Source: CAD feature listing. Evaluate the final solid. Frame: model axes, mm. Face numbers are marked on the shaded views. A direction names the side the tool comes from. Round coordinates to 2 decimals unless told otherwise and drop trailing zeros. Write each loop counter-clockwise with the first axis right and the second up, starting at its lowest first coordinate (ties: lowest second). Pieces come first, ordered by that corner, then holes. Notation, with made-up numbers: (60, 74.5) - (110, 74.5) arc R16 cw to (110, 80.5) - close; hole circle Ø1 at (9, 59). An arc over 180 degrees is marked (long way). Write item = value, one per line. Start each with the question number.
Autodesk Inventor part; units mm, degrees
ref_plane "YZ Plane" through (0, 0, 0) normal (1, 0, 0) x (0, 1, 0)
ref_plane "XZ Plane" through (0, 0, 0) normal (0, 1, 0) x (-1, 0, 0)
ref_plane "XY Plane" through (0, 0, 0) normal (0, 0, 1) x (1, 0, 0)
sketch "Sketch1" plane through (0, 0, 0) normal (1, 0, 0) x (0, 1, 0)
  line L0 (0, 50) -> (0, -50)
  line L1 (0, -50) -> (5, -50)
  line L2 (5, -50) -> (5, -37)
  line L3 (5, -37) -> (17.41, -37)
  line L4 (24, -30.41) -> (24, 30.41)
  line L5 (17.41, 37) -> (5, 37)
  line L6 (5, 37) -> (5, 50)
  line L7 (5, 50) -> (0, 50)
  line L8 (21.5, 11) -> (13.5, 11)
  line L9 (13.5, 11) -> (13.5, -17)
  line L10 (13.5, -17) -> (21.5, -17)
  line L11 (21.5, -17) -> (21.5, 11)
  circle A0 centre (11.9411, 30) radius 4
  circle A1 centre (11.9411, -30) radius 4
  arc A2 (24, 30.41) -> (17.41, 37) centre (17.41, 30.41) ccw
  arc A3 (17.41, -37) -> (24, -30.41) centre (17.41, -30.41) ccw
  point P0 (0, 0)
  point P1 (24, -37)
  point P2 (0, 0)
  dimension "d0" = 100
  dimension "d1" = 5
  dimension "d2" = 13
  dimension "d3" = 13
  dimension "d4" = 19
  dimension "d5" = 28
  dimension "d6" = 26
  dimension "d7" = 8
  dimension "d8" = 2.5
  dimension "d9" = 8
  dimension "d10" = 60
  dimension "d11" = 30
  dimension "d12" = 6.59
extrude "Extrusion1" add sketch "Sketch1" along normal blind 12
sketch "Sketch2" plane through (0, 24, 30.41) normal (0, 1, 0) x (1, 0, 0)
  circle A0 centre (6, 33.41) radius 4
  line L0 (0, -6.59) -> (12, -6.59)
  point P0 (0, 30.41)
  point P1 (6, -6.59)
  dimension "d15" = 40
  dimension "d16" = 8
extrude "Extrusion2" cut sketch "Sketch2" against normal blind 20
sketch "Sketch3" plane through (0, 0, -50) normal (0, -1, 0) x (1, 0, 0)
  line L0 (4, 95) -> (4, 91)
  line L1 (8, 91) -> (8, 95)
  arc A0 (4, 91) -> (8, 91) centre (6, 91) ccw
  arc A1 (8, 95) -> (4, 95) centre (6, 95) ccw
  line L2 (0, 100) -> (12, 100)
  line L3 (0, 100) -> (0, 0)
  line L4 (4, 9) -> (4, 5)
  line L5 (8, 5) -> (8, 9)
  arc A2 (4, 5) -> (8, 5) centre (6, 5) ccw
  arc A3 (8, 9) -> (4, 9) centre (6, 9) ccw
  line L6 (0, 0) -> (12, 0)
  point P0 (0, 50)
  dimension "d19" = 4
  dimension "d20" = 4
  dimension "d21" = 5
  dimension "d22" = 6
  dimension "d23" = 4
  dimension "d24" = 4
  dimension "d25" = 5
extrude "Extrusion3" cut sketch "Sketch3" against normal up to next
sketch "Sketch5" plane through (0, 13.5, 11) normal (0, 1, 0) x (1, 0, 0)
  circle A0 centre (6, 14) radius 4
  circle A1 centre (6, 14) radius 5
  point P0 (0, 11)
  dimension "d28" = 10
extrude "Extrusion4" add sketch "Sketch5" along normal blind 0.5
pattern_linear "Rectangular Pattern1" count 2 spacing 7.5 along (0, 1, 0) of "Extrusion4"
equation "\"d3\" = d2"
properties material "ABS Plastic"
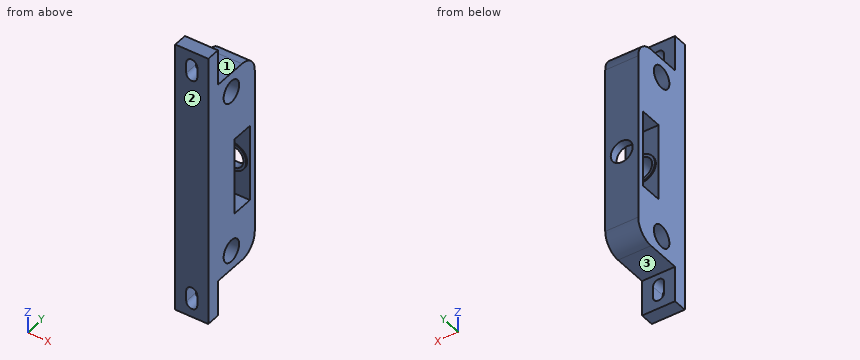
(1) Section C-C (x = 6). Count the separate pieces of the cut face and the enclosed holes in it, plus the area to 3 significant figures.
(2) Contact query for flat-ended pins moving along their axis: P1, Ø13, axis at y = 11.94, z = -30, coming from the -X side; P2, Ø6, axis at x = 8, y = 19, coming from the -Z side; P3, Ø4, axis at x = 6.5, y = 17.5, coming from the +Z side. Output: stop coordinate, or through.
(3) Section D-D (z = 32). Return the cut outline in (x, y).
(4) Section A-A (y = 10.25). Return the cut outline in (x, z), plus the area to 3 significant figures.
(5) Reachability of the marked faces 1, 2 and 3 from +Z, -Z, +X, -X, +Y, -Y: full face, straight path, thin tool, end or side. Return the list, or none.
(6) Section B-B (z = -3). Return the cut outline in (x, y).
(7) Ray query, L1, parallel to Z at x = 5.75, y = 4.5; L2, parallel to Z at x = 6, y = 8.5; L3, parallel to X at y = 22.25, z = -3. Return the intervals inside material, ascending. Write a range as from..to.
Solution:
q1.separate_pieces = 3
q1.enclosed_holes = 2
q1.area = 1,390 mm^2
q2.P1 = 0
q2.P2 = -37
q2.P3 = 37
q3.outline = (0, 0) - (12, 0) - (12, 8.48) - (0, 8.48) - close; (0, 15.41) - (12, 15.41) - (12, 23.81) - (0, 23.81) - close
q4.outline = (0, -37) - (12, -37) - (12, -33.62) - (0, -33.62) - close; (0, -26.38) - (12, -26.38) - (12, 26.38) - (0, 26.38) - close; (0, 33.62) - (12, 33.62) - (12, 37) - (0, 37) - close; hole circle Ø8 at (6, -3)
q4.area = 664 mm^2
q5.face_1 = +Z, +X, -X, +Y
q5.face_2 = +Z, -Z, +X, -X, -Y
q5.face_3 = -Z, +X, -X, +Y
q6.outline = (0, 0) - (12, 0) - (12, 13.5) - (11, 13.5) - (11, 14) - (10, 14) - (10, 4) - (2, 4) - (2, 14) - (1, 14) - (1, 13.5) - (0, 13.5) - close; (0, 21.5) - (1, 21.5) - (1, 21) - (2, 21) - (2, 24) - (0, 24) - close; (10, 21) - (11, 21) - (11, 21.5) - (12, 21.5) - (12, 24) - (10, 24) - close
q7.L1 = -50..-46.98, -39.02..-6.99, 0.99..39.02, 46.98..50
q7.L2 = -37..-32.04, -27.96..-7, 1..27.96, 32.04..37
q7.L3 = 0..2, 10..12
